The drawing under review shows one solid part. Ordinate dimensions are in mm from its lowest x, y, z. Give positions to 0.01 mm unless a question says otherwise; leave off trailing zeros. Order: outer loops, then holes, each group sorted by start corner. A loop starts at its lowest first (then second) coordinate and runs counter-clockwise, first axis right, second up. Notation, with made-up numbers: (75, -33.75) -> (94, -33.75) arc R29 cw to (94, -2.75) -> close; hole circle Ø2 at (55, 51). An arc over 180 degrees is marked (long way). Use a Markdown table: item, result. Add a question column.
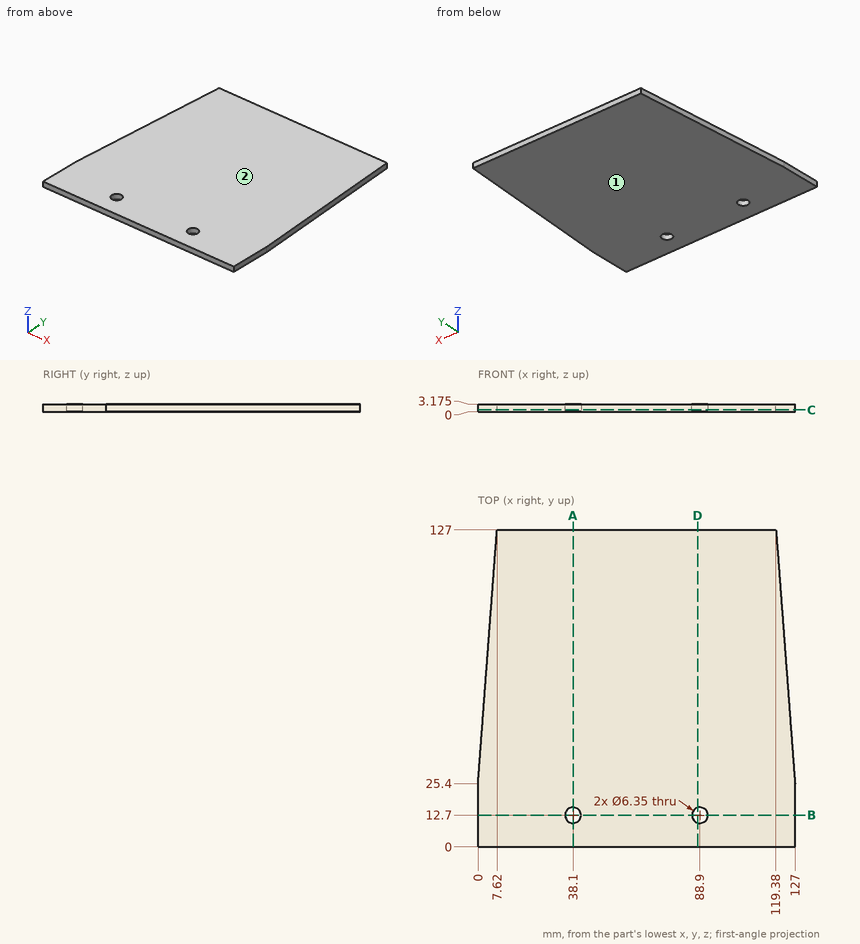
1) The part is to be moulded in two halves that separate along Z. For the marked faces 1 and 2, say which applies: +Z half, -Z half, draft (parallel to the pull), parting line (faces both ways), or undercut.
2) For L1, parallel to Y at x = 38.1, z = 1.5 (3 decimals); L2, parallel to Y at x = 36.5, z = 1; L3, parallel to X at y = 29, z = 0.9, list the stretches that pass through material, from the lowest coordinate up. Write a range as [from, to].
3) Insertion check: pin 1 (8.5 mm diameter, centred on x = 38.1, y = 12.7, fed in from +Z) (3 decimals); pin 2 (1.5 mm diameter, centred on y = 85.5, z = 2.5, fed in from +X); pin 3 (5 mm diameter, centred on x = 88.9, y = 12.7, fed in from +Z). Each pin has a flat end and moves straight along its axis. Give the tip position at first contact, or say it passes through.
4) Add section A-A (x = 38.1). Give the boundary of the cut face in (y, z) (3 decimals), then the cut area to 3 significant figures.
5) Add section B-B (y = 12.7). Give the boundary of the cut face in (x, z) (3 decimals).
6) Add section D-D (x = 88). Give the boundary of the cut face in (y, z) (3 decimals).
7) Add section C-C (z = 0.8). Give the boundary of the cut face in (x, y) (3 decimals), then the cut area to 3 significant figures.
Worked answers:
| question | item | result |
|---|---|---|
| 1 | face 1 | -Z half |
| 1 | face 2 | +Z half |
| 2 | L1 | [0, 9.525], [15.875, 127] |
| 2 | L2 | [0, 9.96], [15.44, 127] |
| 2 | L3 | [0.27, 126.73] |
| 3 | pin 1 | z = 3.175 |
| 3 | pin 2 | x = 122.55 |
| 3 | pin 3 | through |
| 4 | outline | (0, 0) -> (9.525, 0) -> (9.525, 3.175) -> (0, 3.175) -> close; (15.875, 0) -> (127, 0) -> (127, 3.175) -> (15.875, 3.175) -> close |
| 4 | area | 383 mm^2 |
| 5 | outline | (0, 0) -> (34.925, 0) -> (34.925, 3.175) -> (0, 3.175) -> close; (41.275, 0) -> (85.725, 0) -> (85.725, 3.175) -> (41.275, 3.175) -> close; (92.075, 0) -> (127, 0) -> (127, 3.175) -> (92.075, 3.175) -> close |
| 6 | outline | (0, 0) -> (9.655, 0) -> (9.655, 3.175) -> (0, 3.175) -> close; (15.745, 0) -> (127, 0) -> (127, 3.175) -> (15.745, 3.175) -> close |
| 7 | outline | (0, 0) -> (127, 0) -> (127, 25.4) -> (119.38, 127) -> (7.62, 127) -> (0, 25.4) -> close; hole circle Ø6.35 at (38.1, 12.7); hole circle Ø6.35 at (88.9, 12.7) |
| 7 | area | 15,300 mm^2 |
